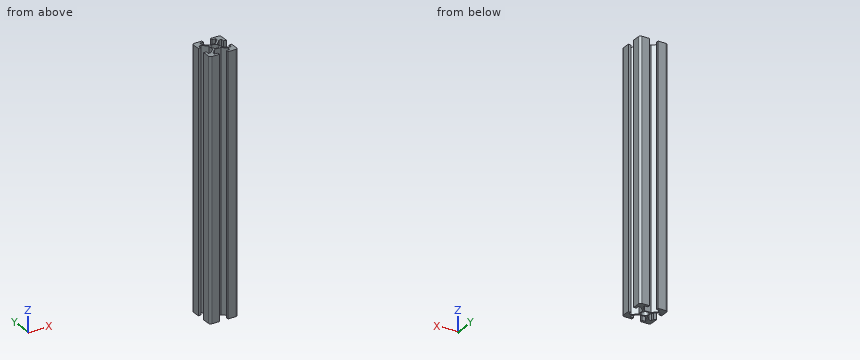
from build123d import *

# Parameters (mm, degrees)
SKETCH_1_R          = 2.5
EXTRUDE_1_DEPTH     = 950
SKETCH_2_W          = 109.948268043
SKETCH_2_H          = 29.443949836
CUT_EXTRUDE_1_DEPTH = 725.86
SKETCH_5_W          = 99.378556311
SKETCH_5_H          = 151.459473896
CUT_EXTRUDE_2_DEPTH = 41


with BuildPart() as part:
    # 草图1 → 凸台-拉伸1 (new body)
    with BuildSketch(Plane.XY):
        with BuildLine():
            Line((-8.2, -3.1), (-10, -3.1))
            Line((-10, -3.1), (-10, -8.5))
            ThreePointArc((-10, -8.5), (-9.560660172, -9.560660172), (-8.5, -10))
            Line((-8.5, -10), (-3.1, -10))
            Line((-3.1, -10), (-3.1, -8.2))
            Line((-3.1, -8.2), (-5.5, -8.2))
            Line((-5.5, -8.2), (-5.5, -6.397050155))
            Line((-5.5, -6.397050155), (-2.202949845, -3.1))
            Line((-2.202949845, -3.1), (2.202949845, -3.1))
            Line((2.202949845, -3.1), (5.5, -6.397050155))
            Line((5.5, -6.397050155), (5.5, -8.2))
            Line((5.5, -8.2), (3.1, -8.2))
            Line((3.1, -8.2), (3.1, -10))
            Line((3.1, -10), (8.5, -10))
            ThreePointArc((8.5, -10), (9.560660172, -9.560660172), (10, -8.5))
            Line((10, -8.5), (10, -3.1))
            Line((10, -3.1), (8.2, -3.1))
            Line((8.2, -3.1), (8.2, -5.5))
            Line((8.2, -5.5), (6.397050155, -5.5))
            Line((6.397050155, -5.5), (3.05412702, -2.157076865))
            Line((3.05412702, -2.157076865), (3.05412702, 2.157076865))
            Line((3.05412702, 2.157076865), (6.397050155, 5.5))
            Line((6.397050155, 5.5), (8.2, 5.5))
            Line((8.2, 5.5), (8.2, 3.1))
            Line((8.2, 3.1), (10, 3.1))
            Line((10, 3.1), (10, 8.5))
            ThreePointArc((10, 8.5), (9.560660172, 9.560660172), (8.5, 10))
            Line((8.5, 10), (3.1, 10))
            Line((3.1, 10), (3.1, 8.2))
            Line((3.1, 8.2), (5.5, 8.2))
            Line((5.5, 8.2), (5.5, 6.397050155))
            Line((5.5, 6.397050155), (2.202949845, 3.1))
            Line((2.202949845, 3.1), (-2.202949845, 3.1))
            Line((-2.202949845, 3.1), (-5.5, 6.397050155))
            Line((-5.5, 6.397050155), (-5.5, 8.2))
            Line((-5.5, 8.2), (-3.1, 8.2))
            Line((-3.1, 8.2), (-3.1, 10))
            Line((-3.1, 10), (-8.5, 10))
            ThreePointArc((-8.5, 10), (-9.560660172, 9.560660172), (-10, 8.5))
            Line((-10, 8.5), (-10, 3.1))
            Line((-10, 3.1), (-8.2, 3.1))
            Line((-8.2, 3.1), (-8.2, 5.5))
            Line((-8.2, 5.5), (-6.397050155, 5.5))
            Line((-6.397050155, 5.5), (-3.05412702, 2.157076865))
            Line((-3.05412702, 2.157076865), (-3.05412702, -2.157076865))
            Line((-3.05412702, -2.157076865), (-6.397050155, -5.5))
            Line((-6.397050155, -5.5), (-8.2, -5.5))
            Line((-8.2, -5.5), (-8.2, -3.1))
        make_face()
        with Locations(Location((0, 0, 0), (0, 0, 180))):
            Circle(SKETCH_1_R, mode=Mode.SUBTRACT)
    extrude(amount=EXTRUDE_1_DEPTH)

    # 草图2 → 切除-拉伸1 (cut)
    with BuildSketch(Plane.XY.offset(950)):
        with Locations((27.511129311, -2.182282155)):
            Rectangle(SKETCH_2_W, SKETCH_2_H)
    extrude(amount=-CUT_EXTRUDE_1_DEPTH, mode=Mode.SUBTRACT)

    # 草图5 → 切除-拉伸2 (cut)
    with BuildSketch(Plane(origin=(0, 0, 0), x_dir=(-1, 0, 0), z_dir=(0, 0, -1))):
        with Locations((35.202237194, -44.495814053)):
            Rectangle(SKETCH_5_W, SKETCH_5_H)
    extrude(amount=-CUT_EXTRUDE_2_DEPTH, mode=Mode.SUBTRACT)


solid = part.part
For this review, take the finished solid that the model builds, in its own axes (mm). Give positions to 0.01 mm unless a question says otherwise; leave off trailing zeros. Order: outer loops, then holes, each group sorted by start corner. A loop starts at its lowest first (then second) coordinate and runs counter-clockwise, first axis right, second up. Notation, with made-up numbers: (-9.5, 20) - (40.5, 20) arc R32 ccw to (40.5, 53) - close; hole circle Ø2 at (-31.5, 51). An arc over 180 degrees is marked (long way). Answer as a JSON object with one key per item and string values. Group by question number.
Item 1: Wall thickness on line 1 along X through (y, z) = (-7.25, 200); line 2 along X through (y, z) = (0.25, 165); line 3 along Y through (x, z) = (0, 107): over which ranges is each line inside the solid? List them lowest first.
Item 2: Clearance check with flat-ended pins moving along their axes: pin 1 Ø1.4 at (y, z) = (-9.5, 127.5) entering from -X; pin 2 Ø1.5 at (x, z) = (-2, 110.5) entering from +Y. State where each tip first meets the part, or that it passes through.
Item 3: Take a section at B-B on x = 0. Give the boundary of the cut face in (y, z).
Item 4: Take a section at A-A on y = 0. Give the boundary of the cut face in (x, z).
Reported:
{
 "1": {"line 1": "-10 to -5.5, 5.5 to 10", "line 2": "-3.05 to -2.49, 2.49 to 3.05", "line 3": "-3.1 to -2.5, 2.5 to 3.1"},
 "2": {"pin 1": "x = -9.97", "pin 2": "y = 3.65"},
 "3": {"outline": "(-3.1, 41) - (-2.5, 41) - (-2.5, 224.14) - (-3.1, 224.14) - close; (2.5, 41) - (3.1, 41) - (3.1, 224.14) - (2.5, 224.14) - close"},
 "4": {"outline": "(-3.05, 41) - (-2.5, 41) - (-2.5, 224.14) - (-3.05, 224.14) - close; (2.5, 41) - (3.05, 41) - (3.05, 224.14) - (2.5, 224.14) - close"}
}
